Can you work these out from the model? Positions are in its coordinate system, mm. Face numbers are marked on the shaded views. A direction names the side the tool comes from. Coordinates: 2 decimals unless noted, no trailing zeros. Loops run counter-clockwise (first coordinate to the right, second up) from the corner with the lowest first, then second, coordinate; pieces in that order, holes last. Notation, with made-up numbers: M 75.25,44 L 99.25,44 A18 ccw 99.25,75 Z; hole C -22,63 d3. An arc over 180 degrees is marked long. Answer as a JSON object with one key per item and string values. Group by question number.
Item 1: Suppose I cut it at A-A (y = 0). Write out the boundary of the cut face in (x, z), then the cut area to 3 significant figures.
Item 2: If I drill on line 1 (Z direction, x = 2, y = 5.25); line 2 (Y direction, x = 0.75, z = 31); line 3 (Z direction, x = -7.5, y = 3.25), over which ranges is the centre line in solid material (lowest first)?
Item 3: Which directions (+Z, -Z, +X, -X, +Y, -Y) give clear straight access to the entire face, cutting with the end or side of a thin tool? Please do the marked faces 1 and 2.
Item 4: I'm going to push flat-ended pins straight in: pin 1 Ø2 at (x, z) = (2.5, 22.5) entering from -Y; pin 2 Ø2 at (x, z) = (1.5, 27.5) entering from -Y; pin 3 Ø1.5 at (x, z) = (-1.5, 22.5) entering from -Y. Where does each tip first touch, or does it pass through?
Item 5: Suppose I cut it at C-C (z = 18). Write out the boundary of the cut face in (x, y).
Autodesk Inventor part; units mm, degrees
ref_plane "YZ Plane" through (0, 0, 0) normal (1, 0, 0) x (0, 1, 0)
ref_plane "XZ Plane" through (0, 0, 0) normal (0, 1, 0) x (-1, 0, 0)
ref_plane "XY Plane" through (0, 0, 0) normal (0, 0, 1) x (1, 0, 0)
sketch "Esboço2" plane through (0, 0, 0) normal (0, 0, 1) x (1, 0, 0)
  circle A0 centre (0, 0) radius 9
  dimension "d10" = 18
extrude "Extrusão1" add sketch "Esboço2" along normal blind 5
sketch "Esboço3" plane through (0, 0, 5) normal (0, 0, 1) x (1, 0, 0)
  circle A0 centre (0, 0) radius 6.5
  dimension "d13" = 13
extrude "Extrusão2" add sketch "Esboço3" along normal blind 4
sketch "Esboço4" plane through (0, 0, 9) normal (0, 0, 1) x (1, 0, 0)
  circle A0 centre (0, 0) radius 3
  dimension "d17" = 6
extrude "Extrusão3" add sketch "Esboço4" along normal blind 25
chamfer "Chanfro2" distance 1 angle 45 1 edges at (-3, 0, 34)
chamfer "Chanfro3" distance 0.5 angle 45 1 edges at (-6.5, 0, 9)
thread "Rosca1"
chamfer "Chanfro5" distance 1 angle 45 1 edges at (-9, 0, 5)
fillet "Arredondamento1" radius 5 1 edges at (-6.5, 0, 5)
properties part number "maniplo" material "Aço, carbono"
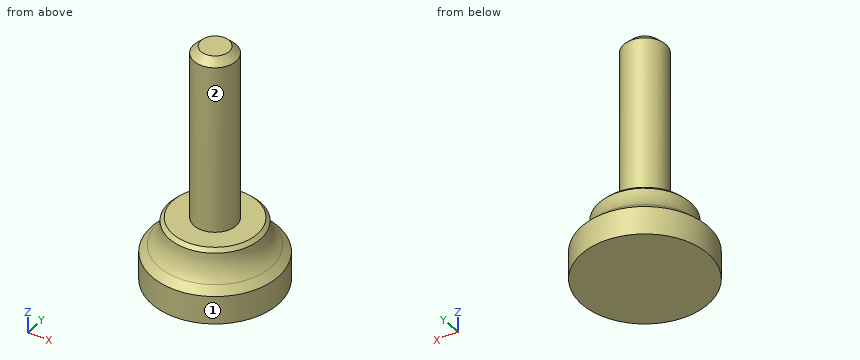
From the geometry:
{
 "1": {"outline": "M -9,0 L 9,0 L 9,4 L 8,5 A5 cw 6.5,8.5 L 6,9 L 3,9 L 3,33 L 2,34 L -2,34 L -3,33 L -3,9 L -6,9 L -6.5,8.5 A5 cw -8,5 L -9,4 Z", "area": "293 mm2"},
 "2": {"line 1": "0 to 9", "line 2": "-2.9 to 2.9", "line 3": "0 to 4.83"},
 "3": {"face 1": "+Z, -Z", "face 2": "+Z"},
 "4": {"pin 1": "y = -2.6", "pin 2": "y = -2.96", "pin 3": "y = -2.9"},
 "5": {"outline": "C 0,0 d6"}
}
